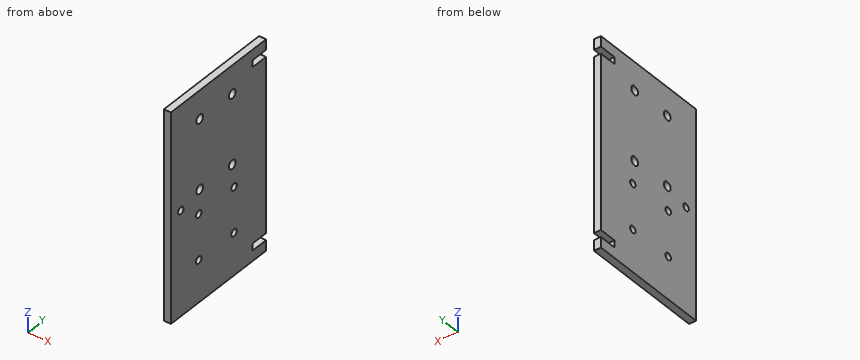
from build123d import *

# Parameters (mm, degrees)
SKETCH_1_W          = 120
SKETCH_1_H          = 70
EXTRUDE_1_DEPTH     = 4
SKETCH_2_R          = 2
SKETCH_2_W          = 4
SKETCH_2_H          = 10
CUT_EXTRUDE_1_DEPTH = 5
SKETCH_3_R          = 2.5
SKETCH_3_R_2        = 2
CUT_EXTRUDE_2_DEPTH = 5


with BuildPart() as part:
    # Эскиз1 → Бобышка-Вытянуть1 (new body)
    with BuildSketch(Plane(origin=(0, 0, 0), x_dir=(0, 0, -1), z_dir=(1, 0, 0))):
        Rectangle(SKETCH_1_W, SKETCH_1_H)
    extrude(amount=EXTRUDE_1_DEPTH)

    # Эскиз2 → Вырез-Вытянуть1 (cut, through all)
    with BuildSketch(Plane(origin=(4, 0, 0), x_dir=(0, 0, -1), z_dir=(1, 0, 0))):
        with Locations((0, -27.660492885)):
            Circle(SKETCH_2_R)
        with Locations((-52, 30)):
            Rectangle(SKETCH_2_W, SKETCH_2_H)
        with Locations((52, 30)):
            Rectangle(SKETCH_2_W, SKETCH_2_H)
    extrude(amount=-CUT_EXTRUDE_1_DEPTH, mode=Mode.SUBTRACT)

    # Эскиз3 → Вырез-Вытянуть2 (cut, through all)
    with BuildSketch(Plane(origin=(4, 0, 0), x_dir=(0, 0, -1), z_dir=(1, 0, 0))):
        with Locations((-43.737507579, 10.172241739)):
            Circle(SKETCH_3_R)
        with Locations((-43.737507579, -13.827758261)):
            Circle(SKETCH_3_R)
        with Locations((-3.737507579, -13.827758261)):
            Circle(SKETCH_3_R)
        with Locations((-3.737507579, 10.172241739)):
            Circle(SKETCH_3_R)
        with Locations((9.8030981, 11.493999532)):
            Circle(SKETCH_3_R_2)
        with Locations((35.8030981, 11.493999532)):
            Circle(SKETCH_3_R_2)
        with Locations((35.8030981, -14.506000468)):
            Circle(SKETCH_3_R_2)
        with Locations((9.8030981, -14.506000468)):
            Circle(SKETCH_3_R_2)
    extrude(amount=-CUT_EXTRUDE_2_DEPTH, mode=Mode.SUBTRACT)


solid = part.part
CAD build for the part. Positions are in the model's coordinates, mm. Round coordinates to 2 decimals unless told otherwise and drop trailing zeros. Order: outer loops, then holes, each group sorted by start corner. A loop starts at its lowest first (then second) coordinate and runs counter-clockwise, first axis right, second up. Notation, with made-up numbers: M -19,6 L 17,6 A31 cw 17,44 Z; hole C 4,68.25 d5. An arc over 180 degrees is marked long. Use one line per item in the form item = value.
Q1. Probe L1, parallel to Z at x = 2.45, y = 26; L2, parallel to Y at x = 1.2, z = 44; L3, parallel to Y at x = 0.6, z = 51. List the from-to ranges inside material, lowest first.
Recorded:
L1 = -60 to -54, -50 to 50, 54 to 60
L2 = -35 to -16.31, -11.34 to 7.69, 12.66 to 35
L3 = -35 to 25
Q2. Flat gauge pin, fed straight in: P1, Ø8, axis at y = -13.83, z = 43.74, coming from the +X side. Where does the tip first touch, or does it go through?
Recorded:
P1 = 4
Q3. Saw through at A-A on z = 0. Give the cut face in (x, y), then the cut area to 3 significant figures.
Recorded:
outline = M 0,-35 L 4,-35 L 4,-29.66 L 0,-29.66 Z; M 0,-25.66 L 4,-25.66 L 4,35 L 0,35 Z
area = 264 mm^2
Q4. Saw through at C-C on z = -35. Give the cut face in (x, y).
Recorded:
outline = M 0,-35 L 4,-35 L 4,-16.34 L 0,-16.34 Z; M 0,-12.67 L 4,-12.67 L 4,9.66 L 0,9.66 Z; M 0,13.33 L 4,13.33 L 4,35 L 0,35 Z
Q5. Saw through at B-B on x = 1.6. State how many separate pieces and enclosed holes the cut face has, then the cut area to 3 significant figures.
Recorded:
separate_pieces = 1
enclosed_holes = 9
area = 8,180 mm^2
